Design review of the part built by this model. Coordinates are the model's own, in mm. Give positions to 0.01 mm unless a question says otherwise; leave off trailing zeros. Write each loop counter-clockwise with the first axis right and the second up, starting at its lowest first coordinate (ties: lowest second). Pieces come first, ordered by that corner, then holes. Notation, with made-up numbers: M 18,-10 L 75,-10 A25 cw 75,11 Z; hole C -29.5,86.5 d2. An arc over 180 degrees is marked long. Use one line per item in the form item = value. Start each with the question number.
from build123d import *

# Parameters (mm, degrees)
SKETCH3_R           = 0.225
BOSS_EXTRUDE1_DEPTH = 13
BOSS_EXTRUDE2_DEPTH = 0.3
FILLET1_R           = 0.25


with BuildPart() as part:
    # Sketch2 → Revolve1 (revolve)
    with BuildSketch(Plane.XY):
        with BuildLine():
            Line((4.5, -0.5), (4, 0))
            Line((4, 0), (0, 0))
            Line((0, 0), (0, -17.2))
            Line((0, -17.2), (4.56, -17.2))
            Line((4.56, -17.2), (4.56, -16.9))
            Line((4.56, -16.9), (4.5, -16.9))
            Line((4.5, -16.9), (4.5, -2.33))
            ThreePointArc((4.5, -2.33), (3.75, -1.58), (4.5, -0.83))
            Line((4.5, -0.83), (4.5, -0.5))
        make_face()
    revolve(axis=Axis((0, 11.579317477, 0), (0, -1, 0)))

    # Sketch3 → Boss-Extrude1 (add)
    with BuildSketch(Plane.XZ.offset(17.2)):
        with Locations((-2.54, 0)):
            Circle(SKETCH3_R)
        with Locations((0, 2.54)):
            Circle(SKETCH3_R)
        with Locations((2.54, 0)):
            Circle(SKETCH3_R)
        with Locations((0, -2.54)):
            Circle(SKETCH3_R)
    extrude(amount=BOSS_EXTRUDE1_DEPTH)

    # Sketch4 → Boss-Extrude2 (add)
    with BuildSketch(Plane.XZ.offset(17.2)):
        with BuildLine():
            Line((2.929134872, 3.494820296), (3.636241653, 4.201927078))
            Line((3.636241653, 4.201927078), (4.201927078, 3.636241653))
            Line((4.201927078, 3.636241653), (3.494820296, 2.929134872))
            ThreePointArc((3.494820296, 2.929134872), (3.224406922, 3.224406922), (2.929134872, 3.494820296))
        make_face()
    extrude(amount=-BOSS_EXTRUDE2_DEPTH)

    # Fillet1
    fillet1_edges = [part.edges().sort_by_distance(p)[0] for p in [
        (4.201927078, -17.05, 3.636241653),
        (3.636241653, -17.05, 4.201927078),
        (2.929134872, -17.05, 3.494820296),
        (3.494820296, -17.05, 2.929134872),
    ]]
    fillet(fillet1_edges, radius=FILLET1_R)

    # Sketch6 → Revolve2 (revolve)
    with BuildSketch(Plane.XY):
        Polygon((0, 0), (0, 45.720209211), (4, 0), align=None)
    revolve(axis=Axis((0, 0, 0), (0, 1, 0)))


solid = part.part
1. We need section B-B (y = 21). State the section outline as (x, z) points, and give its area (3 significant figures).
2. Clearance check with flat-ended pins moving along their axes: pin 1 Ø1.5 at (y, z) = (-4.5, -3) entering from -X; pin 2 Ø4 at (x, y) = (-0.5, -9) entering from -Z; pin 3 Ø5 at (y, z) = (-8, -0.5) entering from -X. State where each tip first meets the part, or that it passes through.
3. We need section A-A (y = -10.5). State the section outline as (x, z) points, and give its area (3 significant figures).
4. To check wall thickness, follow L1, parallel to Y at x = -1.25, z = 4; L2, parallel to Y at x = 4, z = -1; L3, parallel to X at y = 31.5, z = -0.25. State the ranges of each line that lie inside material, in increasing order.
Answer block:
q1.outline = C 0,0 d4.33
q1.area = 14.7 mm^2
q2.pin_1 = -3.9
q2.pin_2 = -4.5
q2.pin_3 = -4.5
q3.outline = C 0,0 d9
q3.area = 63.6 mm^2
q4.L1 = -17.2 to -2.26, -0.9 to -0.19
q4.L2 = -17.2 to -2.23, -0.93 to -0.12
q4.L3 = -1.22 to 1.22
